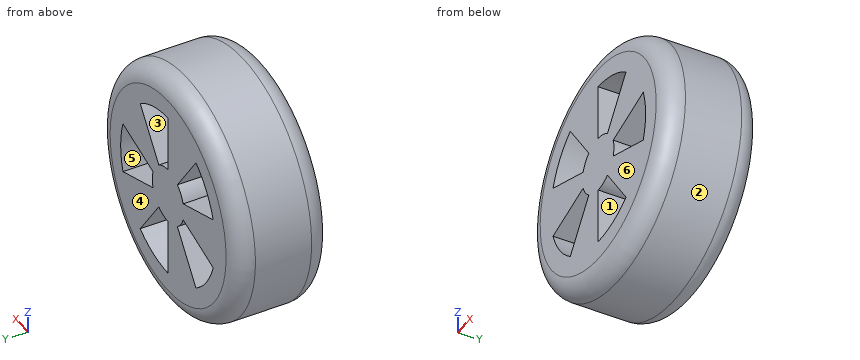
from build123d import *

# Parameters (mm, degrees)
SKETCH_1_R      = 32.5
EXTRUDE_1_DEPTH = 25
FILLET_1_R      = 5
FILLET_2_R      = 5


with BuildPart() as part:
    # 草图1 → 凸台-拉伸1 (new body)
    with BuildSketch(Plane(origin=(0, 0, 0), x_dir=(1, 0, 0), z_dir=(0, 1, 0))):
        with Locations(Location((0, 0, 0), (0, 0, 270))):
            Circle(SKETCH_1_R)
        with BuildLine():
            Line((0, 7.5), (0, 22.5))
            ThreePointArc((0, 22.5), (6.952882373, 21.398771617), (13.225168177, 18.202882373))
            Line((13.225168177, 18.202882373), (4.408389392, 6.067627458))
            ThreePointArc((4.408389392, 6.067627458), (2.317627458, 7.132923872), (0, 7.5))
        make_face(mode=Mode.SUBTRACT)
        with BuildLine():
            Line((7.132923872, 2.317627458), (21.398771617, 6.952882373))
            ThreePointArc((21.398771617, 6.952882373), (22.5, 0), (21.398771617, -6.952882373))
            Line((21.398771617, -6.952882373), (7.132923872, -2.317627458))
            ThreePointArc((7.132923872, -2.317627458), (7.5, 0), (7.132923872, 2.317627458))
        make_face(mode=Mode.SUBTRACT)
        with BuildLine():
            Line((4.408389392, -6.067627458), (13.225168177, -18.202882373))
            ThreePointArc((13.225168177, -18.202882373), (6.952882373, -21.398771617), (0, -22.5))
            Line((0, -22.5), (0, -7.5))
            ThreePointArc((0, -7.5), (2.317627458, -7.132923872), (4.408389392, -6.067627458))
        make_face(mode=Mode.SUBTRACT)
        with BuildLine():
            Line((-4.408389392, -6.067627458), (-13.225168177, -18.202882373))
            ThreePointArc((-13.225168177, -18.202882373), (-18.202882373, -13.225168177), (-21.398771617, -6.952882373))
            Line((-21.398771617, -6.952882373), (-7.132923872, -2.317627458))
            ThreePointArc((-7.132923872, -2.317627458), (-6.067627458, -4.408389392), (-4.408389392, -6.067627458))
        make_face(mode=Mode.SUBTRACT)
        with BuildLine():
            Line((-7.132923872, 2.317627458), (-21.398771617, 6.952882373))
            ThreePointArc((-21.398771617, 6.952882373), (-18.202882373, 13.225168177), (-13.225168177, 18.202882373))
            Line((-13.225168177, 18.202882373), (-4.408389392, 6.067627458))
            ThreePointArc((-4.408389392, 6.067627458), (-6.067627458, 4.408389392), (-7.132923872, 2.317627458))
        make_face(mode=Mode.SUBTRACT)
    extrude(amount=EXTRUDE_1_DEPTH)

    # 圆角1
    fillet_1_edges = [part.edges().sort_by_distance(p)[0] for p in [
        (0, 25, -32.5),
    ]]
    fillet(fillet_1_edges, radius=FILLET_1_R)

    # 圆角2
    fillet_2_edges = [part.edges().sort_by_distance(p)[0] for p in [
        (0, 0, -32.5),
    ]]
    fillet(fillet_2_edges, radius=FILLET_2_R)


solid = part.part
Verification items for the finished model (mm, model axes). Face numbers are marked on the shaded views. A direction names the side the tool comes from. Give positions to 0.01 mm unless a question says otherwise; leave off trailing zeros. Write each loop counter-clockwise with the first axis right and the second up, starting at its lowest first coordinate (ties: lowest second). Pieces come first, ordered by that corner, then holes.
(1) Access from +Z, -Z, +X, -X, +Y, -Y to the whole of each face (thin tool, end or side, straight path). Record for the marked faces 5 and 6.
(2) Gauge pin test, flat ends, axial feed: pin 1 (4.5 mm diameter, centred on y = 10.5, z = -12, fed in from +X); pin 2 (1.5 mm diameter, centred on x = 14, y = 5, fed in from +Z); pin 3 (5 mm diameter, centred on y = 16, z = 2.5, fed in from -X). Record the tip position at first contact, or that the pin passes through.
(3) Material ranges on line 1 (Z direction, x = 5, y = 3.75); line 2 (X direction, y = 19.5, z = -12.5); line 3 (X direction, y = 5, z = 10.5), recorded low to high.
(4) Cross-section at C-C (y = 2.5). Enter the section's corners in (x, z).
(5) Cross-section at B-B (y = 10.75). Enter the section's corners in (x, z).
(6) Cross-section at A-A (z = 0). Enter the section's corners in (x, y).
(7) Mould release check, pull along Z, two halves, no side actions. Record for the marked faces 1, 2, 3 and 4: +Z half, -Z half, draft (parallel to the pull), parting line (faces both ways), or undercut.
(8) Cross-section at D-D (z = 10). State how many separate pieces and enclosed holes the cut face has, plus the area to 3 significant figures.
Worked out:
1. face 5: +Y, -Y
1. face 6: +Z, -Z, +X, -X, -Y
2. pin 1: stops at x = 31
2. pin 2: stops at z = 29.68
2. pin 3: stops at x = -32.5
3. line 1: z = -31.95 to -21.94, -6.88 to 6.88, 21.94 to 31.95
3. line 2: x = -30 to -18.71, -9.08 to 0, 9.08 to 30
3. line 3: x = -30.76 to -19.9, -7.63 to 0, 7.63 to 30.76
4. outline: circle Ø63.66 at (0, 0); hole (-21.4, -6.95) arc R22.5 ccw to (-13.23, -18.2) - (-4.41, -6.07) arc R7.5 cw to (-7.13, -2.32) - close; hole (-21.4, 6.95) - (-7.13, 2.32) arc R7.5 cw to (-4.41, 6.07) - (-13.23, 18.2) arc R22.5 ccw to start; hole (0, -22.5) arc R22.5 ccw to (13.23, -18.2) - (4.41, -6.07) arc R7.5 cw to (0, -7.5) - close; hole (0, 7.5) arc R7.5 cw to (4.41, 6.07) - (13.23, 18.2) arc R22.5 ccw to (0, 22.5) - close; hole (7.13, -2.32) - (21.4, -6.95) arc R22.5 ccw to (21.4, 6.95) - (7.13, 2.32) arc R7.5 cw to start
5. outline: circle Ø65 at (0, 0); hole (-21.4, -6.95) arc R22.5 ccw to (-13.23, -18.2) - (-4.41, -6.07) arc R7.5 cw to (-7.13, -2.32) - close; hole (-21.4, 6.95) - (-7.13, 2.32) arc R7.5 cw to (-4.41, 6.07) - (-13.23, 18.2) arc R22.5 ccw to start; hole (0, -22.5) arc R22.5 ccw to (13.23, -18.2) - (4.41, -6.07) arc R7.5 cw to (0, -7.5) - close; hole (0, 7.5) arc R7.5 cw to (4.41, 6.07) - (13.23, 18.2) arc R22.5 ccw to (0, 22.5) - close; hole (7.13, -2.32) - (21.4, -6.95) arc R22.5 ccw to (21.4, 6.95) - (7.13, 2.32) arc R7.5 cw to start
6. outline: (-32.5, 5) arc R5 ccw to (-27.5, 0) - (7.5, 0) - (7.5, 25) - (-27.5, 25) arc R5 ccw to (-32.5, 20) - close; (22.5, 0) - (27.5, 0) arc R5 ccw to (32.5, 5) - (32.5, 20) arc R5 ccw to (27.5, 25) - (22.5, 25) - close
7. face 1: undercut
7. face 2: parting line
7. face 3: undercut
7. face 4: draft
8. separate pieces: 3
8. enclosed holes: 0
8. area: 1,020 mm2
